```python
from build123d import *

# Parameters (mm, degrees)
MODEL_R             = 3
BOSS_EXTRUDE1_DEPTH = 6


with BuildPart() as part:
    # Model → Boss-Extrude1 (new body)
    with BuildSketch(Plane.XY):
        with BuildLine():
            Line((122.81162835, 8.788979227), (21.34180525, 8.788979227))
            Line((21.34180525, 8.788979227), (21.081967495, 45.003500256))
            ThreePointArc((21.081967495, 45.003500256), (72.0767168, 96.735308544), (123.071466105, 45.003500256))
            Line((123.071466105, 45.003500256), (122.81162835, 8.788979227))
        make_face()
        with Locations((72.0767168, 45.735308544)):
            Circle(MODEL_R, mode=Mode.SUBTRACT)
        Polygon((49.802853193, 68.009172151), (56.697144309, 74.903463268), (52.808057013, 78.792550564), (39.01947478, 65.003968331), (42.908562076, 61.114881035), align=None, mode=Mode.SUBTRACT)
        Polygon((49.802853193, 23.461444937), (56.697144309, 16.56715382), (52.808057013, 12.678066524), (39.01947478, 26.466648757), (42.908562076, 30.355736053), align=None, mode=Mode.SUBTRACT)
        Polygon((94.350580407, 68.009172151), (101.244871524, 61.114881035), (105.13395882, 65.003968331), (91.345376587, 78.792550564), (87.456289291, 74.903463268), align=None, mode=Mode.SUBTRACT)
        Polygon((94.350580407, 23.461444937), (101.244871524, 30.355736053), (105.13395882, 26.466648757), (91.345376587, 12.678066524), (87.456289291, 16.56715382), align=None, mode=Mode.SUBTRACT)
    extrude(amount=BOSS_EXTRUDE1_DEPTH)


solid = part.part
```
CAD build for the part. Positions are in the model's coordinates, mm. A direction names the side the tool comes from. Round coordinates to 2 decimals unless told otherwise and drop trailing zeros. Loops run counter-clockwise (first coordinate to the right, second up) from the corner with the lowest first, then second, coordinate; pieces in that order, holes last. Notation, with made-up numbers: M -27.75,-11.5 L 13.25,-11.5 A12 ccw 13.25,2.5 Z; hole C -26,53 d11. An arc over 180 degrees is marked long. Return JSON: item names as keys, results as strings. Group by question number.
(1) Drop a flat-ended pin along its axis: P1, Ø9.5, axis at x = 72.08, y = 45.74, coming from the -Z side. Give the stop position or say it passes through.
(2) Saw through at A-A, the plane y = 63. List the corners of the cut face in (x, z).
(3) Wall check: probe 1 along Y at (x, z) = (48, 5.55); probe 2 along X at (y, z) = (64, 0.45); probe 3 along X at (y, z) = (67, 4). Give the ranges that are in metal, low to high. Write a range as [from, to].
(4) Mould opens along X. For faces 3 (the flat face through (73, 53, 0)), 4 (the flat face through (46.01, 19.476, 2.958)), 5 (the cylindrical face through (70.945, 96.723, 2.958)) say: +X half, -X half, draft (parallel to the pull), parting line (faces both ways), or undercut.
(5) Tool access for faces 1 (the flat face through (40.937, 63.087, 2.958)), 2 (the flat face through (73, 53, 6)): list every direction of +Z, -Z, +X, -X, +Y, -Y with a clear straight run to the whole face (end or side of a thin tool).
(6) Saw through at C-C, the plane x = 31.5. List the corners of the cut face in (y, z).
(7) Saw through at B-B, the plane z = 1.5. List the corners of the cut face in (x, y), and give its area (3 significant figures).
(8) Saw through at D-D, the plane y = 73. List the corners of the cut face in (x, z), and give its area (3 significant figures).
Answer list:
{
 "1": {"P1": "z = 0"},
 "2": {"outline": "M 24.09,0 L 41.02,0 L 41.02,6 L 24.09,6 Z; M 44.79,0 L 99.36,0 L 99.36,6 L 44.79,6 Z; M 103.13,0 L 120.07,0 L 120.07,6 L 103.13,6 Z"},
 "3": {"probe 1": "[8.79, 17.49], [25.26, 66.21], [73.98, 90.69]", "probe 2": "[24.46, 40.02], [45.79, 98.36], [104.13, 119.69]", "probe 3": "[25.72, 41.02], [48.79, 95.36], [103.14, 118.43]"},
 "4": {"face 3": "draft", "face 4": "undercut", "face 5": "parting line"},
 "5": {"face 1": "+Z, -Z", "face 2": "+Z, +X, -X, +Y, -Y"},
 "6": {"outline": "M 8.79,0 L 76.63,0 L 76.63,6 L 8.79,6 Z"},
 "7": {"outline": "M 21.08,45 L 21.34,8.79 L 122.81,8.79 L 123.07,45 A51 ccw long Z; hole M 39.02,26.47 L 52.81,12.68 L 56.7,16.57 L 42.91,30.36 Z; hole M 39.02,65 L 42.91,61.11 L 56.7,74.9 L 52.81,78.79 Z; hole C 72.08,45.74 d6; hole M 87.46,16.57 L 91.35,12.68 L 105.13,26.47 L 101.24,30.36 Z; hole M 87.46,74.9 L 101.24,61.11 L 105.13,65 L 91.35,78.79 Z", "area": "7,390 mm2"},
 "8": {"outline": "M 28.98,0 L 47.02,0 L 47.02,6 L 28.98,6 Z; M 54.79,0 L 89.36,0 L 89.36,6 L 54.79,6 Z; M 97.14,0 L 115.18,0 L 115.18,6 L 97.14,6 Z", "area": "424 mm2"}
}
